Here's how the part is built. I have some questions about the finished solid (model axes, mm). Round coordinates to 2 decimals unless told otherwise and drop trailing zeros. Order: outer loops, then holes, each group sorted by start corner. A loop starts at its lowest first (then second) coordinate and runs counter-clockwise, first axis right, second up. Notation, with made-up numbers: M 79,75.25 L 109,75.25 A26 ccw 109,108.25 Z; hole C 2,83 d11. An arc over 180 degrees is marked long. Write item = value, one per line. Start each with the question number.
Item 1: I want a section at A-A, the plane z = -14.5. State how many separate pieces and enclosed holes the cut face has, plus the area to 3 significant figures.
Item 2: I want a section at B-B, the plane x = 151. List the corners of the cut face in (y, z) for me, plus the area to 3 significant figures.
Item 3: Please list where these lines run through material, in increasing order: L1, parallel to Z at x = 27, y = 0; L2, parallel to Z at x = 386, y = 1; L3, parallel to Y at x = 19.05, z = -10.
Item 4: I want a section at D-D, the plane y = -16. List the corners of the cut face in (x, z) for me, plus the area to 3 significant figures.
Item 5: I'm going to push flat-ended pins straight in: P1, Ø10, axis at x = 218.5, z = 12, coming from the -Y side; P2, Ø8.5, axis at y = 0, z = 0, coming from the +X side; P3, Ø1.9, axis at x = 19.05, y = 0, coming from the -Z side; P4, Ø2, axis at x = 258, z = 17, coming from the -Y side. Where does each tip first touch, or does it pass through?
Item 6: I want a section at C-C, the plane y = 9. List the corners of the cut face in (x, z) for me.
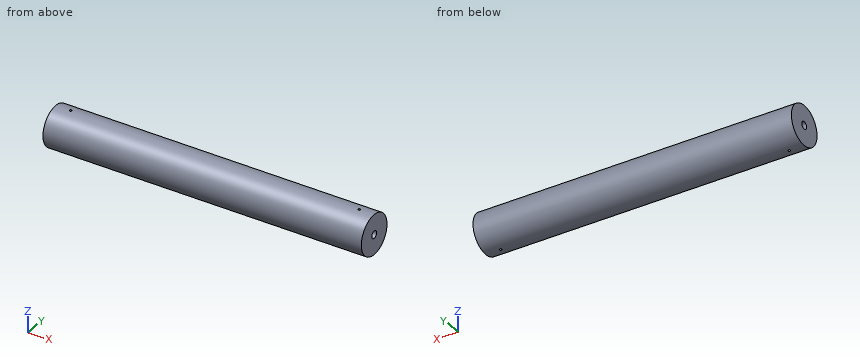
```python
from build123d import *

# Parameters (mm, degrees)
F0_R     = 25.4
F1_DEPTH = 406.4
F3_D     = 9.525
F3_DEPTH = 38.1
F3_TIP   = 2.8615986981
F5_D     = 9.525
F5_DEPTH = 38.1
F5_TIP   = 2.8615986981
F6_R     = 1.5875
F7_DEPTH = 25.4
F9_DEPTH = 31.75


with BuildPart() as f1:
    # F0 (on Right) → F1 (new body)
    with BuildSketch(Plane.YZ):
        Circle(F0_R)
    extrude(amount=F1_DEPTH)

    # F3
    with Locations(Plane.YZ.offset(406.4)):
        with Locations((0, 0)):
            Hole(F3_D / 2, depth=F3_DEPTH)
            with Locations((0, 0, -(F3_DEPTH + F3_TIP / 2))):  # 118° drill point
                Cone(0, F3_D / 2, F3_TIP, mode=Mode.SUBTRACT)

    # F5
    with Locations(Plane(origin=(0, 0, 0), x_dir=(0, -1, 0), z_dir=(-1, 0, 0))):
        with Locations((0, 0)):
            Hole(F5_D / 2, depth=F5_DEPTH)
            with Locations((0, 0, -(F5_DEPTH + F5_TIP / 2))):  # 118° drill point
                Cone(0, F5_D / 2, F5_TIP, mode=Mode.SUBTRACT)


with BuildPart() as f7:
    # F6 (on Top) → F7 (new body, symmetric)
    with BuildSketch(Plane.XY):
        with Locations((19.05, 0)):
            Circle(F6_R)
    extrude(amount=F7_DEPTH, both=True)


with BuildPart() as f1_1:
    add(f1.part)

    # F8: cut F7
    add(f7.part, mode=Mode.SUBTRACT)


with BuildPart() as f9:
    # F6 (on Top) → F9 (new body, symmetric)
    with BuildSketch(Plane.XY):
        with Locations((387.35, 0)):
            Circle(F6_R)
    extrude(amount=F9_DEPTH, both=True)


with BuildPart() as f1_2:
    add(f1_1.part)

    # F10: cut F9
    add(f9.part, mode=Mode.SUBTRACT)


solid = f1_2.part
```
Filled in:
q1.separate_pieces = 1
q1.enclosed_holes = 2
q1.area = 16,900 mm^2
q2.outline = C 0,0 d50.8
q2.area = 2,030 mm^2
q3.L1 = -25.4 to -4.76, 4.76 to 25.4
q3.L2 = -25.38 to -4.66, 4.66 to 25.38
q3.L3 = -23.35 to -1.59, 1.59 to 23.35
q4.outline = M 0,-19.73 L 406.4,-19.73 L 406.4,19.73 L 0,19.73 Z
q4.area = 16,000 mm^2
q5.P1 = -24.42
q5.P2 = 367.99
q5.P3 = through
q5.P4 = -19.73
q6.outline = M 0,-23.75 L 406.4,-23.75 L 406.4,23.75 L 0,23.75 Z
